For this review, take the finished solid that the model builds, in its own axes (mm). Give positions to 0.01 mm unless a question says otherwise; leave off trailing zeros. Loops run counter-clockwise (first coordinate to the right, second up) from the corner with the lowest first, then second, coordinate; pieces in that order, holes last. Notation, with made-up numbers: (-30, -24.75) -> (-24, -24.75) arc R12 cw to (-24, -19.75) -> close; hole circle Ø7 at (87, -29.5). An arc over 180 degrees is marked (long way). Write each question's results on one line, items separated by ' | '. Start each with the question number.
Autodesk Inventor part; units mm, degrees
ref_plane "YZ Plane" through (0, 0, 0) normal (1, 0, 0) x (0, 1, 0)
ref_plane "XZ Plane" through (0, 0, 0) normal (0, 1, 0) x (-1, 0, 0)
ref_plane "XY Plane" through (0, 0, 0) normal (0, 0, 1) x (1, 0, 0)
sketch "Sketch1" plane through (0, 0, 0) normal (0, 1, 0) x (-1, 0, 0)
  circle A0 centre (0, 0) radius 63.5
  dimension "d0" = 127
extrude "Extrusion1" add sketch "Sketch1" along normal blind 12.7
sketch "Sketch2" plane through (0, 12.7, 0) normal (0, 1, 0) x (1, 0, 0)
  point P0 (0, 0)
  point P1 (26.4475, 5.8254)
hole "Hole1" at (0, 12.7, 0) direction (0, -1, 0) diameter 7.1374 end through all
sketch "Sketch3" plane through (0, 0, 0) normal (0, -1, 0) x (1, 0, 0)
  circle A0 centre (0, 0) radius 3.5687
  line L0 (6.4231, 0) -> (3.2116, -5.5626)
  line L1 (3.2116, -5.5626) -> (-3.2116, -5.5626)
  line L2 (-3.2116, -5.5626) -> (-6.4231, 0)
  line L3 (-6.4231, 0) -> (-3.2116, 5.5626)
  line L4 (-3.2116, 5.5626) -> (3.2116, 5.5626)
  line L5 (3.2116, 5.5626) -> (6.4231, 0)
  dimension "d10" = 11.1252
extrude "Extrusion2" cut sketch "Sketch3" against normal blind 4.3688 contours A0 | L0 L1 L2 L3 L4 L5
chamfer "Chamfer1" distance 0.508 angle 45 6 edges at (4.8174, 0, 2.7813) (0, 0, 5.5626) (-4.8174, 0, 2.7813) (-4.8174, 0, -2.7813) (0, 0, -5.5626) (4.8174, 0, -2.7813)
sketch "Sketch4" plane through (0, 0, 0) normal (0, 0, 1) x (1, 0, 0)
  line L0 (-63.5, 0) -> (-63.5, 12.7)
  line L1 (-63.5, 3.81) -> (-62.23, 3.81)
  line L2 (-62.23, 3.81) -> (-62.23, 1.905)
  line L3 (-62.23, 1.905) -> (-63.5, 1.905)
  line L4 (-63.5, 1.905) -> (-63.5, 3.81)
  line L5 (-63.5, 10.795) -> (-62.23, 10.795)
  line L6 (-62.23, 10.795) -> (-62.23, 8.89)
  line L7 (-62.23, 8.89) -> (-63.5, 8.89)
  line L8 (-63.5, 8.89) -> (-63.5, 10.795)
  line L9 (-63.5, 6.35) -> (-70.565, 6.35)
  line L10 (0, 0) -> (0, 18.3077)
  dimension "d16" = 1.27
  dimension "d17" = 1.905
  dimension "d18" = 5.08
revolve "Revolution1" cut sketch "Sketch4" angle 360 about axis through (0, 0, 0) along (0, 1, 0)
properties part number "Piston Head"
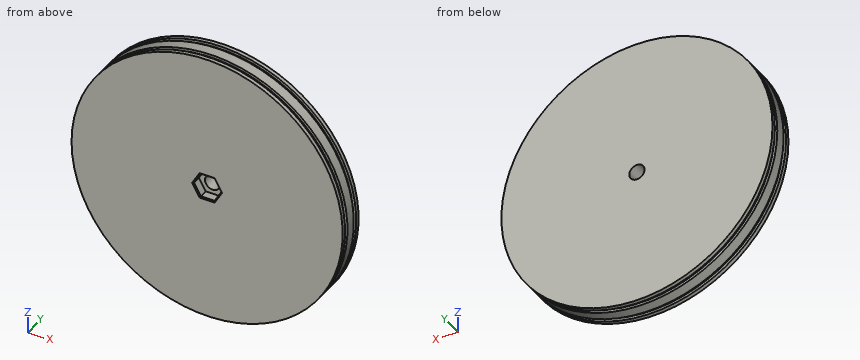
1. For pin 1 Ø3 at (x, y) = (1, 2.5) entering from -Z; pin 2 Ø2 at (y, z) = (9.5, -27) entering from -X; pin 3 Ø1.5 at (x, y) = (29.5, 7.5) entering from +Z, all flat-tipped, find the tip position at first contact; note any pin that passes through.
2. We need section B-B (z = -41). Write out the cut boundary in (x, y) (3 decimals).
3. We need section C-C (x = -16.5). Write out the cut boundary in (y, z) (3 decimals).
4. Wall thickness on L1, parallel to Z at x = 0, y = 10.5; L2, parallel to Z at x = 0, y = 8.5; L3, parallel to X at y = 11.75, z = -12.5: over which ranges is each line inside the solid? List them lowest first.
Response:
1) pin 1: stops at z = -63.5 | pin 2: stops at x = -57.84 | pin 3: stops at z = 56.62
2) outline: (-48.49, 0) -> (48.49, 0) -> (48.49, 1.905) -> (46.814, 1.905) -> (46.814, 3.81) -> (48.49, 3.81) -> (48.49, 8.89) -> (46.814, 8.89) -> (46.814, 10.795) -> (48.49, 10.795) -> (48.49, 12.7) -> (-48.49, 12.7) -> (-48.49, 10.795) -> (-46.814, 10.795) -> (-46.814, 8.89) -> (-48.49, 8.89) -> (-48.49, 3.81) -> (-46.814, 3.81) -> (-46.814, 1.905) -> (-48.49, 1.905) -> close
3) outline: (0, -61.319) -> (1.905, -61.319) -> (1.905, -60.003) -> (3.81, -60.003) -> (3.81, -61.319) -> (8.89, -61.319) -> (8.89, -60.003) -> (10.795, -60.003) -> (10.795, -61.319) -> (12.7, -61.319) -> (12.7, 61.319) -> (10.795, 61.319) -> (10.795, 60.003) -> (8.89, 60.003) -> (8.89, 61.319) -> (3.81, 61.319) -> (3.81, 60.003) -> (1.905, 60.003) -> (1.905, 61.319) -> (0, 61.319) -> close
4) L1: z = -62.23 to -3.57, 3.57 to 62.23 | L2: z = -63.5 to -3.57, 3.57 to 63.5 | L3: x = -62.26 to 62.26
